```python
from build123d import *

# Parameters (mm, degrees)
F0_W      = 184.15
F0_H      = 50.8
F1_DEPTH  = 8.128
F3_D      = 5.1054
F6_D      = 4.9784
F7_W      = 76.2
F7_H      = 9.525
F8_DEPTH  = 8.129
F9_SIZE   = 9.525
F10_SIZE  = 2.54
F11_R     = 2.4892
F12_DEPTH = 4.064
F13_SIZE  = 4.06399


# Not quite as in the source:
# - a fillet or chamfer is up to 0.001 mm smaller than in the source, because OpenCascade refuses the exact size


with BuildPart() as f1:
    # F0 (on Top) → F1 (new body)
    with BuildSketch(Plane.XY):
        Rectangle(F0_W, F0_H)
    extrude(amount=F1_DEPTH)

    # F3 (through all)
    with Locations(Plane.XY.offset(8.128)):
        with Locations((-60.325, 12.7), (-76.2, -12.7), (-44.45, -12.7)):
            Hole(F3_D / 2)

    # F6 (through all)
    with Locations(Plane.XY.offset(8.128)):
        with Locations((79.375, 12.7), (79.375, -12.7)):
            Hole(F6_D / 2)

    # F7 (on face) → F8 (cut, through all)
    with BuildSketch(Plane.XY.offset(8.128)):
        Polygon((66.675, 25.4), (-47.625, 25.4), (-34.925, 12.7), (53.975, 12.7), align=None)
        with Locations((15.875, -4.7625)):
            Rectangle(F7_W, F7_H)
    extrude(amount=-F8_DEPTH, mode=Mode.SUBTRACT)

    # F9
    f9_edges = [f1.edges().sort_by_distance(p)[0] for p in [
        (-92.075, -25.4, 4.064),
        (-92.075, 25.4, 4.064),
        (92.075, -25.4, 4.064),
        (92.075, 25.4, 4.064),
    ]]
    chamfer(f9_edges, length=F9_SIZE)

    # F10
    f10_edges = [f1.edges().sort_by_distance(p)[0] for p in [
        (-22.225, 0, 4.064),
        (-22.225, -9.525, 4.064),
        (53.975, 0, 4.064),
        (53.975, -9.525, 4.064),
    ]]
    chamfer(f10_edges, length=F10_SIZE)

    # F11 (on face) → F12 (cut)
    with BuildSketch(Plane.XY.offset(8.128)):
        Polygon((82.55, 25.4), (66.675, 25.4), (66.675, -25.4), (82.55, -25.4), (92.075, -15.875), (92.075, 15.875), align=None)
        with Locations((79.375, -12.7)):
            Circle(F11_R, mode=Mode.SUBTRACT)
        with Locations((79.375, 12.7)):
            Circle(F11_R, mode=Mode.SUBTRACT)
    extrude(amount=-F12_DEPTH, mode=Mode.SUBTRACT)

    # F13 (size 4.064 in the source; OpenCascade refuses exactly that, so slightly less here)
    f13_edges = [f1.edges().sort_by_distance(p)[0] for p in [
        (66.675, 0, 4.064),
    ]]
    chamfer(f13_edges, length=F13_SIZE)


solid = f1.part
```
Part model, mm, in its own coordinate system. A direction names the side the tool comes from. Coordinates: 2 decimals unless noted, no trailing zeros. Order: outer loops, then holes, each group sorted by start corner. A loop starts at its lowest first (then second) coordinate and runs counter-clockwise, first axis right, second up. Notation, with made-up numbers: (52.5, -28) - (100.5, -28) arc R26 ccw to (100.5, 3) - close; hole circle Ø8 at (28, 36.25). An arc over 180 degrees is marked (long way). Return JSON: item names as keys, results as strings. Group by question number.
Item 1: Cut at A-A (x = -76.2). List the corners of the cut face in (y, z).
Item 2: Which spindle directions (+Z, -Z, +X, -X, +Y, -Y) get a long thin tool onto all of the face, cutting with end or side? Do faces 4 (the face through (81, 0, 4.064)), 5 (the face through (53.975, -5, 4)), 6 (the face through (-41.364, 19.139, 4.121)). Say none if no direction does.
Item 3: Cut at C-C (z = 1.5). List the corners of the cut face in (x, y) (3 decimals), plus the area to 3 significant figures.
Item 4: Pin check, flat tips, straight feed: pin 1 (10.5 mm diameter, centred on x = 83, y = 4.5, fed in from +Z); pin 2 (2.5 mm diameter, centred on x = 5.5, z = 3.5, fed in from +Y); pin 3 (3 mm diameter, centred on x = -60.325, y = 12.7, fed in from -Z); pin 4 (8 mm diameter, centred on x = -76.2, y = -12.7, fed in from +Z). Stop position of each tip, or through.
Item 5: Cut at D-D (y = -12.7). State how many separate pieces and enclosed holes the cut face has, plus the area to 3 significant figures.
Item 6: Pull direction X, two halves, no side cores. Call faces 1 (the face through (-13.8, 0.4, 8.128)), 2 (the face through (87.38, -20.57, 2)), 3 (the face through (-57.775, 12.812, 4.007)): pulls with the +X half, pulls with the -X half, needs draft (parallel to the pull), parting line crosses it, or undercut.
Item 7: Drill centre lines: probe 1 along Y at (x, z) = (22.5, 2) (3 decimals); probe 2 along X at (y, z) = (-3.5, 3) (3 decimals); probe 3 along X at (y, z) = (20, 2) (3 decimals). Where is each one in solid material? Low to high. Write a range as from..to.
Check values:
{
 "1": {"outline": "(-25.4, 0) - (-15.25, 0) - (-15.25, 8.13) - (-25.4, 8.13) - close; (-10.15, 0) - (25.4, 0) - (25.4, 8.13) - (-10.15, 8.13) - close"},
 "2": {"face 4": "+Z, +X, +Y, -Y", "face 5": "+Z, -Z", "face 6": "+Z, -Z, +Y"},
 "3": {"outline": "(-92.075, -15.875) - (-82.55, -25.4) - (82.55, -25.4) - (92.075, -15.875) - (92.075, 15.875) - (82.55, 25.4) - (66.675, 25.4) - (53.975, 12.7) - (-34.925, 12.7) - (-47.625, 25.4) - (-82.55, 25.4) - (-92.075, 15.875) - close; hole circle Ø5.105 at (-76.2, -12.7); hole circle Ø5.105 at (-60.325, 12.7); hole circle Ø5.105 at (-44.45, -12.7); hole (-22.225, -6.985) - (-19.685, -9.525) - (51.435, -9.525) - (53.975, -6.985) - (53.975, -2.54) - (51.435, 0) - (-19.685, 0) - (-22.225, -2.54) - close; hole circle Ø4.978 at (79.375, -12.7); hole circle Ø4.978 at (79.375, 12.7)", "area": "7,070 mm2"},
 "4": {"pin 1": "stops at z = 4.06", "pin 2": "stops at y = 12.7", "pin 3": "passes through", "pin 4": "stops at z = 8.13"},
 "5": {"separate pieces": "4", "enclosed holes": "0", "area": "1,300 mm2"},
 "6": {"face 1": "needs draft", "face 2": "pulls with the +X half", "face 3": "undercut"},
 "7": {"probe 1": "y = -25.4..-9.525, 0..12.7", "probe 2": "x = -92.075..-22.225, 53.975..92.075", "probe 3": "x = -87.95..-42.225, 61.275..87.95"}
}
